```python
from build123d import *
from build123d.topology import SkipClean

# Parameters (mm, degrees)
SKETCH_1_R          = 3
SKETCH_1_R_2        = 1.5
EXTRUDE_1_DEPTH     = 2.5
SKETCH_2_R          = 4.75
EXTRUDE_2_DEPTH     = 5
CUT_EXTRUDE_START   = -3
SKETCH_3_R          = 3
CUT_EXTRUDE_1_DEPTH = 3
SKETCH_4_R          = 1.5
CUT_EXTRUDE_2_DEPTH = 3


with BuildPart() as part:
    # 草图1 → 凸台-拉伸1 (new body)
    with BuildSketch(Plane(origin=(0, 0, 0), x_dir=(1, 0, 0), z_dir=(0, 1, 0))):
        with BuildLine():
            Line((0.296875, 4.740713579), (20.21875, 3.493157374))
            ThreePointArc((20.21875, 3.493157374), (23.5, 0), (20.21875, -3.493157374))
            Line((20.21875, -3.493157374), (0.296875, -4.740713579))
            ThreePointArc((0.296875, -4.740713579), (-4.75, 0), (0.296875, 4.740713579))
        make_face()
        with Locations(Location((0, 0, 0), (0, 0, 270))):
            Circle(SKETCH_1_R, mode=Mode.SUBTRACT)
        with Locations(Location((20, 0, 0), (0, 0, 270))):
            Circle(SKETCH_1_R_2, mode=Mode.SUBTRACT)
    extrude(amount=EXTRUDE_1_DEPTH)

    # 草图2 → 凸台-拉伸2 (add)
    with SkipClean():  # the faces are left unmerged after this step: merging them gives an invalid solid
        with BuildSketch(Plane(origin=(0, 2.5, 0), x_dir=(1, 0, 0), z_dir=(0, 1, 0))):
            with Locations(Location((0, 0, 0), (0, 0, 86.416678302))):
                Circle(SKETCH_2_R)
        extrude(amount=EXTRUDE_2_DEPTH)

    # 草图3 → 切除-拉伸1 (cut)
    with SkipClean():  # the faces are left unmerged after this step: merging them gives an invalid solid
        with BuildSketch(Plane(origin=(0, 7.5, 0), x_dir=(1, 0, 0), z_dir=(0, 1, 0)).offset(CUT_EXTRUDE_START)):
            with Locations(Location((0, 0, 0), (0, 0, 270))):
                Circle(SKETCH_3_R)
        extrude(amount=CUT_EXTRUDE_1_DEPTH, mode=Mode.SUBTRACT)

    # 草图4 → 切除-拉伸2 (cut)
    with SkipClean():  # the faces are left unmerged after this step: merging them gives an invalid solid
        with BuildSketch(Plane.XZ.offset(-2.5)):
            with Locations(Location((0, 0, 0), (0, 0, 270))):
                Circle(SKETCH_4_R)
        extrude(amount=-CUT_EXTRUDE_2_DEPTH, mode=Mode.SUBTRACT)


solid = part.part
```
Can you work these out from the model? Positions are in its coordinate system, mm. A direction names the side the tool comes from. Give positions to 0.01 mm unless a question says otherwise; leave off trailing zeros. Loops run counter-clockwise (first coordinate to the right, second up) from the corner with the lowest first, then second, coordinate; pieces in that order, holes last. Notation, with made-up numbers: M 0.5,37 L 22.5,37 A25 cw 22.5,59 Z; hole C 34.25,32.25 d8. An arc over 180 degrees is marked long. Use CSV: the item, a comma, the result in double quotes. Start each with the question number.
1. If I drill on L1, parallel to X at y = 0.6, z = 0; L2, parallel to X at y = 3.1, z = 0; L3, parallel to Y at x = 15, z = -3, over which ranges is the centre line in solid material (lowest first)?
2. If we mould it in two halves opening along X, with no side actions, what happens to faces 4 (the face through (12, 2.5, 0)), 5 (the face through (-1.3, 4.5, 1.3)), 6 (the face through (23.5, 1.2, -0.1))? For each: released by +X, released by -X, zero draft, split by the parting line, or undercut.
3. Imagine slicing it at D-D, the plane y = 6.25. Write out the boundary of the cut face in (x, z).
4. Imagine slicing it at B-B, the plane z = 0. Write out the boundary of the cut face in (x, y).
5. On a 3-axis mill with a long thin cutter (end or side, diameter ignored), from which of +Z, -Z, +X, -X, +Y, -Y can I reach the whole of each face in a straight line? I mean faces 1 (the face through (0.9, 5.98, 2.86)), 2 (the face through (0.9, 1.23, 2.86)), 3 (the face through (10.118, 1.232, -4.126)). Say none if no direction works.
6. For P1, Ø1.8, axis at x = 1, z = 0, coming from the +Y side; P2, Ø1.5, axis at x = -0.5, y = 1, coming from the -Z side; P3, Ø3, axis at y = 5.5, z = -1, coming from the +X side; P4, Ø3.5, axis at x = 0, z = 0, coming from the -Y side, each with a flat end and sliding along its axis, tell me the tip position at first contact or that it passes through.
7. Imagine slicing it at C-C, the plane y = 1.75. Write out the boundary of the cut face in (x, z).
8. Imagine slicing it at A-A, the plane x = 0. Write out the boundary of the cut face in (y, z), plus the area to 4 significant figures.
Response values:
1,L1,"-4.75 to -3, 3 to 18.5, 21.5 to 23.5"
1,L2,"-4.75 to -1.5, 1.5 to 4.75"
1,L3,"0 to 2.5"
2,face 4,"zero draft"
2,face 5,"undercut"
2,face 6,"released by +X"
3,outline,"C 0,0 d9.5; hole C 0,0 d6"
4,outline,"M -4.75,0 L -3,0 L -3,2.5 L -1.5,2.5 L -1.5,4.5 L -3,4.5 L -3,7.5 L -4.75,7.5 Z; M 1.5,2.5 L 3,2.5 L 3,0 L 18.5,0 L 18.5,2.5 L 4.75,2.5 L 4.75,7.5 L 3,7.5 L 3,4.5 L 1.5,4.5 Z; M 21.5,0 L 23.5,0 L 23.5,2.5 L 21.5,2.5 Z"
5,face 1,"+Y"
5,face 2,"-Y"
5,face 3,"-Z, +X, +Y, -Y"
6,P1,"y = 4.5"
6,P2,"z = -4.75"
6,P3,"x = 4.75"
6,P4,"y = 2.5"
7,outline,"M 0.3,-4.74 L 20.22,-3.49 A3.5 ccw 20.22,3.49 L 0.3,4.74 A4.75 ccw long Z; hole C 0,0 d6; hole C 20,0 d3"
8,outline,"M 0,-4.75 L 7.5,-4.75 L 7.5,-3 L 4.5,-3 L 4.5,-1.5 L 2.5,-1.5 L 2.5,-3 L 0,-3 Z; M 0,3 L 2.5,3 L 2.5,1.5 L 4.5,1.5 L 4.5,3 L 7.5,3 L 7.5,4.75 L 0,4.75 Z"
8,area,"32.25 mm^2"
